The model under review builds one solid part; all positions refer to its coordinate system, in mm. A direction names the side the tool comes from. Round coordinates to 2 decimals unless told otherwise and drop trailing zeros. Write each loop counter-clockwise with the first axis right and the second up, starting at its lowest first coordinate (ties: lowest second). Pieces come first, ordered by that corner, then holes. Notation, with made-up numbers: (5.25, 42.5) -> (37.25, 42.5) arc R13 ccw to (37.25, 67.5) -> close; hole circle Ø6 at (50, 19). An arc over 180 degrees is marked (long way). Answer as a JSON object with one key per item and string values. Group by question number.
1) We need section C-C, the plane y = 7.5. Write out the cut boundary in (x, z).
2) Mouldability with a two-part tool opening along Z and no side actions: class faces 1 (the cylindrical face through (0.16, 16.5, 5.42)), 2 (the flat face through (0, -2, 26)), 3 (the flat face through (-2, -3, 16)) as pulls with the +Z half, pulls with the -Z half, needs draft (parallel to the pull), parting line crosses it, or undercut.
3) Insertion check: pin 1 Ø2.5 at (x, z) = (17.5, 5.5) entering from +Y; pin 2 Ø7.5 at (x, z) = (14, 16.5) entering from +Y; pin 3 Ø12 at (x, z) = (0, 17.41) entering from +Y. Each pin has a flat end and moves straight along its axis. Give the tip position at first contact, or say it passes through.
4) We need section A-A, the plane z = 5.5. Write out the cut boundary in (x, y).
5) Machinability: for faces 4 (the flat face through (-11.913, 4, 18)), 5 (the flat face through (-17, 9, 13)), 6 (the flat face through (15, 9, 13)), 7 (the cylindrical face through (-19.6, 0.13, 6.16)), 8 (the cylindrical face through (0.49, -1.48, 21.13)), which of the approach directions +Z, -Z, +X, -X, +Y, -Y give a long, thin tool a straight path to every point of the face, cutting with its end or side? Answer none if there is none.
6) We need section D-D, the plane x = 17.5. Write out the cut boundary in (y, z).
7) We need section B-B, the plane x = 0. Write out the cut boundary in (y, z).
8) To check wall thickness, follow probe 1 along Z at (x, y) = (17.5, -0.5); probe 2 along X at (y, z) = (0.75, 14.5); probe 3 along Z at (x, y) = (0, -7.5). State the ranges of each line that lie inside material, in increasing order. Write a range as [from, to].
from build123d import *

# Parameters (mm, degrees)
F0_R      = 6.25
F1_DEPTH  = 11
F2_R      = 2.2
F3_DEPTH  = 18.001
F5_DEPTH  = 15
F6_R      = 3.75
F6_R_2    = 2.2
F7_DEPTH  = 3
F7_FACE_R = 2.2
F8_DEPTH  = 9.001


with BuildPart() as f1:
    # F0 (on Top) → F1 (new body)
    with BuildSketch(Plane.XY):
        with BuildLine():
            Line((-7.5, 9), (-22.5, 9))
            Line((-22.5, 9), (-22.5, -9))
            Line((-22.5, -9), (22.5, -9))
            Line((22.5, -9), (22.5, 9))
            Line((22.5, 9), (7.5, 9))
            ThreePointArc((7.5, 9), (0, 1.5), (-7.5, 9))
        make_face()
        with BuildLine():
            ThreePointArc((7.5, 9), (0, 16.5), (-7.5, 9))
            ThreePointArc((-7.5, 9), (0, 1.5), (7.5, 9))
        make_face()
        with Locations((0, 9)):
            Circle(F0_R, mode=Mode.SUBTRACT)
    extrude(amount=F1_DEPTH)

    # F2 (on face) → F3 (cut, through all)
    with BuildSketch(Plane(origin=(0, 9, 0), x_dir=(-1, 0, 0), z_dir=(0, 1, 0))):
        with Locations((17.5, 5.5)):
            Circle(F2_R)
        with Locations((-17.5, 5.5)):
            Circle(F2_R)
    extrude(amount=-F3_DEPTH, mode=Mode.SUBTRACT)

    # F4 (on face) → F5 (join)
    with BuildSketch(Plane.XY.offset(11)):
        Polygon((-11.913064, 9), (-22.5, 9), (-22.5, -9), (22.5, -9), (22.5, 9), (10.984777, 9), (10.984777, 0), (-11.913064, 0), align=None)
    extrude(amount=F5_DEPTH)

    # F6 (on face) → F7 (cut)
    with BuildSketch(Plane(origin=(0, 0, 0), x_dir=(-1, 0, 0), z_dir=(0, 1, 0))):
        with Locations((0, 17.412443)):
            Circle(F6_R)
        with Locations((0, 17.412443)):
            Circle(F6_R_2, mode=Mode.SUBTRACT)
    extrude(amount=-F7_DEPTH, mode=Mode.SUBTRACT)

    # F7_face (on face) → F8 (cut, through all)
    with BuildSketch(Plane(origin=(0, 0, 17.412443), x_dir=(-1, 0, 0), z_dir=(0, 1, 0))):
        Circle(F7_FACE_R)
    extrude(amount=-F8_DEPTH, mode=Mode.SUBTRACT)


solid = f1.part
Here are the results:
{
 "1": {"outline": "(-22.5, 0) -> (-6.07, 0) -> (-6.07, 11) -> (-11.91, 11) -> (-11.91, 26) -> (-22.5, 26) -> close; (6.07, 0) -> (22.5, 0) -> (22.5, 26) -> (10.98, 26) -> (10.98, 11) -> (6.07, 11) -> close; hole circle Ø4.4 at (-17.5, 5.5); hole circle Ø4.4 at (17.5, 5.5)"},
 "2": {"face 1": "needs draft", "face 2": "pulls with the +Z half", "face 3": "undercut"},
 "3": {"pin 1": "passes through", "pin 2": "stops at y = 9", "pin 3": "stops at y = 0"},
 "4": {"outline": "(-22.5, -9) -> (-19.7, -9) -> (-19.7, 9) -> (-22.5, 9) -> close; (-15.3, -9) -> (15.3, -9) -> (15.3, 9) -> (7.5, 9) arc R7.5 ccw to (-7.5, 9) -> (-15.3, 9) -> close; (19.7, -9) -> (22.5, -9) -> (22.5, 9) -> (19.7, 9) -> close; hole circle Ø12.5 at (0, 9)"},
 "5": {"face 4": "+Z, +Y", "face 5": "+Z, -Z, -X, +Y", "face 6": "+Z, -Z, +X, +Y", "face 7": "+Y, -Y", "face 8": "+Y"},
 "6": {"outline": "(-9, 0) -> (9, 0) -> (9, 3.3) -> (-9, 3.3) -> close; (-9, 7.7) -> (9, 7.7) -> (9, 26) -> (-9, 26) -> close"},
 "7": {"outline": "(-9, 0) -> (2.75, 0) -> (2.75, 11) -> (0, 11) -> (0, 13.66) -> (-3, 13.66) -> (-3, 15.21) -> (-9, 15.21) -> close; (-9, 19.61) -> (-3, 19.61) -> (-3, 21.16) -> (0, 21.16) -> (0, 26) -> (-9, 26) -> close; (15.25, 0) -> (16.5, 0) -> (16.5, 11) -> (15.25, 11) -> close"},
 "8": {"probe 1": "z = [0, 3.3], [7.7, 26]", "probe 2": "x = [-22.5, -11.91], [10.98, 22.5]", "probe 3": "z = [0, 15.21], [19.61, 26]"}
}
